Input: part model. Units: mm. Frame: model coordinates. Face numbers are marked on the shaded views. A direction names the side the tool comes from. Round coordinates to 2 decimals unless told otherwise and drop trailing zeros. Loops run counter-clockwise (first coordinate to the right, second up) from the corner with the lowest first, then second, coordinate; pieces in that order, holes last.
1) Section B-B, the plane x = 25.5. Return loops of the section in (y, z).
2) Draft query along X for the marked faces 3 and 4. Return one class per face: pulls with the +X half, pulls with the -X half, needs draft (parallel to the pull), parting line crosses it, or undercut.
3) First-contact query: pin 1 (12 mm diameter, centred on x = 14.5, z = 24.5, fed in from +Y); pin 2 (0.6 mm diameter, centred on x = 19.5, y = 2, fed in from +Z); pin 3 (3.5 mm diameter, centred on y = -3, z = 64, fed in from +X); pin 4 (10 mm diameter, centred on x = 26, z = 29.5, fed in from +Y). Flat tips, straight axial feed; report the tip coordinate or a pass-through.
4) Access query for the marked faces 1 and 2. Directions: +Z, -Z, +X, -X, +Y, -Y. A direction counts if a zero-diameter tool reaches every point of the face in a straight line with its end or side. Return the directions, or none.
5) Section A-A, the plane z = 42. Return loops of the section in (x, y).
6) Section C-C, the plane y = -7.25. Return loops of the section in (x, z), and give its area (3 significant figures).
7) Ray query, line 1 along Y through (x, z) = (25.75, 42); line 2 along Y through (x, z) = (27, 52.5). Return the intervals inside material, ascending.
8) Section D-D, the plane x = 14.5. Return loops of the section in (y, z), and give its area (3 significant figures).
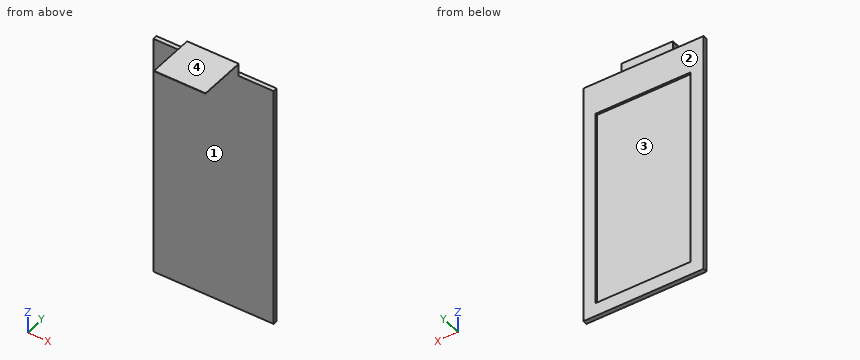
from build123d import *

# Parameters (mm, degrees)
BOSS_EXTRUDE1_DEPTH = 1.5
SKETCH2_W           = 29.2
SKETCH2_H           = 59.2
BOSS_EXTRUDE2_DEPTH = 1.05
SKETCH3_W           = 12.5
SKETCH3_H           = 14.3
BOSS_EXTRUDE3_DEPTH = 0.1
SKETCH4_W           = 12.5
SKETCH4_H           = 3.5
BOSS_EXTRUDE4_DEPTH = 0.2
SKETCH5_W           = 12.5
SKETCH5_H           = 11.4
BOSS_EXTRUDE5_DEPTH = 0.1
SKETCH6_W           = 12.5
SKETCH6_H           = 0.3
CUT_EXTRUDE1_DEPTH  = 11.3
CUT_EXTRUDE2_DEPTH  = 1.5
SKETCH10_W          = 23.000919901
SKETCH10_H          = 48.161967413
CUT_EXTRUDE3_DEPTH  = 0.5


with BuildPart() as part:
    # Sketch1 → Boss-Extrude1 (new body)
    with BuildSketch(Plane(origin=(0, 0, 0), x_dir=(1, 0, 0), z_dir=(0, 1, 0))):
        with BuildLine():
            Line((3.25, 0), (26.95, 0))
            ThreePointArc((26.95, 0), (29.248097039, -0.951902961), (30.2, -3.25))
            Line((30.2, -3.25), (30.2, -61.75))
            ThreePointArc((30.2, -61.75), (29.248097039, -64.048097039), (26.95, -65))
            Line((26.95, -65), (3.25, -65))
            ThreePointArc((3.25, -65), (0.951902961, -64.048097039), (0, -61.75))
            Line((0, -61.75), (0, -3.25))
            ThreePointArc((0, -3.25), (0.951902961, -0.951902961), (3.25, 0))
        make_face()
    extrude(amount=BOSS_EXTRUDE1_DEPTH)

    # Sketch2 → Boss-Extrude2 (add)
    with BuildSketch(Plane(origin=(0, 1.5, 0), x_dir=(1, 0, 0), z_dir=(0, 1, 0))):
        with Locations((15.1, -32.5)):
            Rectangle(SKETCH2_W, SKETCH2_H)
    extrude(amount=BOSS_EXTRUDE2_DEPTH)

    # Sketch3 → Boss-Extrude3 (add)
    with BuildSketch(Plane(origin=(0, 1.5, 0), x_dir=(1, 0, 0), z_dir=(0, 1, 0))):
        with Locations((14.89, -69.25)):
            Rectangle(SKETCH3_W, SKETCH3_H)
    extrude(amount=BOSS_EXTRUDE3_DEPTH)

    # Sketch4 → Boss-Extrude4 (add)
    with BuildSketch(Plane(origin=(0, 1.6, 0), x_dir=(1, 0, 0), z_dir=(0, 1, 0))):
        with Locations((14.89, -74.65)):
            Rectangle(SKETCH4_W, SKETCH4_H)
    extrude(amount=BOSS_EXTRUDE4_DEPTH)

    # Sketch5 → Boss-Extrude5 (add)
    with BuildSketch(Plane.XY.offset(65)):
        with Locations((14.89, -4.2)):
            Rectangle(SKETCH5_W, SKETCH5_H)
    extrude(amount=BOSS_EXTRUDE5_DEPTH)

    # Sketch6 → Cut-Extrude1 (cut)
    with BuildSketch(Plane.XY.offset(76.4)):
        with Locations((14.89, 1.65)):
            Rectangle(SKETCH6_W, SKETCH6_H)
    extrude(amount=-CUT_EXTRUDE1_DEPTH, mode=Mode.SUBTRACT)

    # Sketch8 → Cut-Extrude2 (cut)
    with BuildSketch(Plane.XZ):
        with BuildLine():
            Line((21.14, 65), (8.64, 65))
            Line((8.64, 65), (3.25, 65))
            ThreePointArc((3.25, 65), (0.951902961, 64.048097039), (0, 61.75))
            Line((0, 61.75), (0, 3.25))
            ThreePointArc((0, 3.25), (0.951902961, 0.951902961), (3.25, 0))
            Line((3.25, 0), (26.95, 0))
            ThreePointArc((26.95, 0), (29.248097039, 0.951902961), (30.2, 3.25))
            Line((30.2, 3.25), (30.2, 61.75))
            ThreePointArc((30.2, 61.75), (29.248097039, 64.048097039), (26.95, 65))
            Line((26.95, 65), (21.14, 65))
        make_face()
    extrude(amount=-CUT_EXTRUDE2_DEPTH, mode=Mode.SUBTRACT)

    # Sketch10 → Cut-Extrude3 (cut)
    with BuildSketch(Plane(origin=(0, 2.55, 0), x_dir=(1, 0, 0), z_dir=(0, 1, 0))):
        with Locations((15.222162275, -30.236639689)):
            Rectangle(SKETCH10_W, SKETCH10_H)
    extrude(amount=-CUT_EXTRUDE3_DEPTH, mode=Mode.SUBTRACT)


solid = part.part
Final values:
1. outline: (1.5, 2.9) - (2.55, 2.9) - (2.55, 6.16) - (2.05, 6.16) - (2.05, 54.32) - (2.55, 54.32) - (2.55, 62.1) - (1.5, 62.1) - close
2. face 3: undercut
2. face 4: needs draft
3. pin 1: stops at y = 2.05
3. pin 2: stops at z = 62.1
3. pin 3: stops at x = 21.14
3. pin 4: stops at y = 2.55
4. face 1: -Z, +X, -X, -Y
4. face 2: +Z, -Z, +X, -X, +Y
5. outline: (0.5, 1.5) - (29.7, 1.5) - (29.7, 2.55) - (26.72, 2.55) - (26.72, 2.05) - (3.72, 2.05) - (3.72, 2.55) - (0.5, 2.55) - close
6. outline: (8.64, 65) - (21.14, 65) - (21.14, 65.1) - (8.64, 65.1) - close
6. area: 1.25 mm2
7. line 1: y = 1.5 to 2.05
7. line 2: y = 1.5 to 2.55
8. outline: (-9.9, 65) - (1.5, 65) - (1.5, 2.9) - (2.55, 2.9) - (2.55, 6.16) - (2.05, 6.16) - (2.05, 54.32) - (2.55, 54.32) - (2.55, 62.1) - (1.6, 62.1) - (1.6, 65.1) - (-9.9, 65.1) - close
8. area: 39.5 mm2
